```python
from build123d import *

# Parameters (mm, degrees)
CYLINDER003_R               = 2.3
CYLINDER003_DEPTH           = 40
CYLINDER003_PITCH_ANGLE     = 90
CYLINDER003_PLACEMENT_ANGLE = 7e-06
CYLINDER002_R               = 2.3
CYLINDER002_DEPTH           = 10
CYLINDER001_R               = 2.3
CYLINDER001_DEPTH           = 10
BOX002_W                    = 1.4
BOX002_H                    = 20
BOX002_DEPTH                = 20
CYLINDER_R                  = 8
CYLINDER_DEPTH              = 30
CYLINDER_ROLL_ANGLE         = -90
BOX001_W                    = 25
BOX001_H                    = 16
BOX001_DEPTH                = 36
BOX_W                       = 48
BOX_H                       = 16
BOX_DEPTH                   = 8
FILLET_R                    = 2
FILLET001_R                 = 2


with BuildPart() as cylinder003:
    # Cylinder003 → Cylinder003 (new body)
    with BuildSketch(Plane.XY):
        Circle(CYLINDER003_R)
    extrude(amount=CYLINDER003_DEPTH)


with BuildPart() as cylinder003_1:
    # Cylinder003 pitch: moved
    add(cylinder003.part.rotate(Axis((0, 0, 0), (0, 1, 0)), CYLINDER003_PITCH_ANGLE))


with BuildPart() as cylinder003_2:
    # Cylinder003 placement: moved
    add(cylinder003_1.part.moved(Location((3.687557, 7.912557, 39.313553))).rotate(Axis((3.687557, 7.912557, 39.313553), (0, 0, 1)), CYLINDER003_PLACEMENT_ANGLE))


with BuildPart() as cylinder002:
    # Cylinder002 → Cylinder002 (new body)
    with BuildSketch(Plane(origin=(42.25, 7.8, -0.597231), x_dir=(1, 0, 0), z_dir=(0, 0, 1))):
        Circle(CYLINDER002_R)
    extrude(amount=CYLINDER002_DEPTH)


with BuildPart() as cylinder001:
    # Cylinder001 → Cylinder001 (new body)
    with BuildSketch(Plane(origin=(5.75, 7.8, -0.597231), x_dir=(1, 0, 0), z_dir=(0, 0, 1))):
        Circle(CYLINDER001_R)
    extrude(amount=CYLINDER001_DEPTH)


with BuildPart() as box002:
    # Box002 → Box002 (new body)
    with BuildSketch(Plane(origin=(23.074221, -2.91866, 34.283958), x_dir=(1, 0, 0), z_dir=(0, 0, 1))):
        with Locations((0.7, 10)):
            Rectangle(BOX002_W, BOX002_H)
    extrude(amount=BOX002_DEPTH)


with BuildPart() as cylinder:
    # Cylinder → Cylinder (new body)
    with BuildSketch(Plane.XY):
        Circle(CYLINDER_R)
    extrude(amount=CYLINDER_DEPTH)


with BuildPart() as cylinder_1:
    # Cylinder roll: moved
    add(cylinder.part.rotate(Axis((0, 0, 0), (1, 0, 0)), CYLINDER_ROLL_ANGLE))


with BuildPart() as cylinder_2:
    # Cylinder placement: moved
    add(cylinder_1.part.moved(Location((23.7403, -8.80917, 27))))


with BuildPart() as box001:
    # Box001 → Box001 (new body)
    with BuildSketch(Plane(origin=(11.5, 0, 8), x_dir=(1, 0, 0), z_dir=(0, 0, 1))):
        with Locations((12.5, 8)):
            Rectangle(BOX001_W, BOX001_H)
    extrude(amount=BOX001_DEPTH)


with BuildPart() as fillet001:
    # Box → Box (new body)
    with BuildSketch(Plane.XY):
        with Locations((24, 8)):
            Rectangle(BOX_W, BOX_H)
    extrude(amount=BOX_DEPTH)

    # Fusion: union Box001
    add(box001.part)

    # Cut: cut Cylinder
    add(cylinder_2.part, mode=Mode.SUBTRACT)

    # Cut001: cut Box002
    add(box002.part, mode=Mode.SUBTRACT)

    # Cut002: cut Cylinder001
    add(cylinder001.part, mode=Mode.SUBTRACT)

    # Cut003: cut Cylinder002
    add(cylinder002.part, mode=Mode.SUBTRACT)

    # Cut004: cut Cylinder003
    add(cylinder003_2.part, mode=Mode.SUBTRACT)

    # Fillet
    fillet_edges = [fillet001.edges().sort_by_distance(p)[0] for p in [
        (36.5, 8, 44),
    ]]
    fillet(fillet_edges, radius=FILLET_R)

    # Fillet001
    fillet001_edges = [fillet001.edges().sort_by_distance(p)[0] for p in [
        (11.5, 8, 44),
    ]]
    fillet(fillet001_edges, radius=FILLET001_R)


solid = fillet001.part
```
The listing builds one solid part. Answer for the finished solid, in the listing's coordinates (mm). A direction names the side the tool comes from. Round coordinates to 2 decimals unless told otherwise and drop trailing zeros. Loops run counter-clockwise (first coordinate to the right, second up) from the corner with the lowest first, then second, coordinate; pieces in that order, holes last. Notation, with made-up numbers: (-21, 41.5) -> (27, 41.5) arc R18 cw to (27, 74.5) -> close; hole circle Ø5 at (-28.75, 82). An arc over 180 degrees is marked (long way). Use one line per item in the form item = value.
1. A tool of negligible diameter and unlimited length cuts with its end or side. For faces 1 (the flat face through (4, 10, 8)), 2 (the flat face through (24.474, 10, 41)), 3 (the cylindrical face through (39.952, 7.901, 3.944)), 4 (the flat face through (41, 10, 8)), from which of +Z, -Z, +X, -X, +Y, -Y can it reach the whole face along a straight path? Write none if from no direction.
Answer key:
face_1 = +Z, -X, +Y, -Y
face_2 = +Z, +Y, -Y
face_3 = +Z, -Z
face_4 = +Z, +X, +Y, -Y
2. The part is cut by section C-C on y = 15. Determine the outline of the cut face in (x, z).
Answer key:
outline = (0, 0) -> (48, 0) -> (48, 8) -> (36.5, 8) -> (36.5, 42) arc R2 ccw to (34.5, 44) -> (24.47, 44) -> (24.47, 34.97) arc R8 cw (long way) to (23.07, 34.97) -> (23.07, 44) -> (13.5, 44) arc R2 ccw to (11.5, 42) -> (11.5, 8) -> (0, 8) -> close
3. The part is cut by section D-D on z = 5. Determine the outline of the cut face in (x, y), and give its area (3 significant figures).
Answer key:
outline = (0, 0) -> (48, 0) -> (48, 16) -> (0, 16) -> close; hole circle Ø4.6 at (5.75, 7.8); hole circle Ø4.6 at (42.25, 7.8)
area = 735 mm²
4. For a pull along Y with two mould halves and no side action, classify faces 5 (the cylindrical face through (30.4, 7.03, 37.19)), 6 (the flat face through (11.5, 8, 25)), 7 (the cylindrical face through (17.21, 7.03, 37.19)), 8 (the flat face through (24, 0, 17)) as released by +Y, released by -Y, zero draft, split by the parting line, or undercut.
Answer key:
face_5 = undercut
face_6 = zero draft
face_7 = undercut
face_8 = released by -Y
5. Find the intervals of material crossed by probe 1 along X at (y, z) = (11.75, 35); probe 2 along X at (y, z) = (8.25, 6); probe 3 along X at (y, z) = (9.5, 27), in increasing order. Write a range as [from, to].
Answer key:
probe_1 = [11.5, 23.07], [24.47, 36.5]
probe_2 = [0, 3.49], [8.01, 39.99], [44.51, 48]
probe_3 = [11.5, 15.74], [31.74, 36.5]
6. Flat-ended cylindrical pins translate along their axes: pin 1 Ø9 at (x, y) = (7.5, 9.5) entering from +Z; pin 2 Ø3 at (y, z) = (7.5, 37) entering from +X; pin 3 Ø3 at (x, y) = (42.25, 7.8) entering from +Z; pin 4 Ø6 at (y, z) = (4.5, 25) entering from -X. Find the tip coordinate at first contact, or state that the pin passes through.
Answer key:
pin_1 = 43.32
pin_2 = 36.5
pin_3 = through
pin_4 = 11.5
7. The part is cut by section B-B on z = 27. Determine the outline of the cut face in (x, y), and give its area (3 significant figures).
Answer key:
outline = (11.5, 0) -> (15.74, 0) -> (15.74, 16) -> (11.5, 16) -> close; (31.74, 0) -> (36.5, 0) -> (36.5, 16) -> (31.74, 16) -> close
area = 144 mm²
8. The part is cut by section A-A on x = 5.75. Determine the outline of the cut face in (y, z).
Answer key:
outline = (0, 0) -> (5.5, 0) -> (5.5, 8) -> (0, 8) -> close; (10.1, 0) -> (16, 0) -> (16, 8) -> (10.1, 8) -> close
